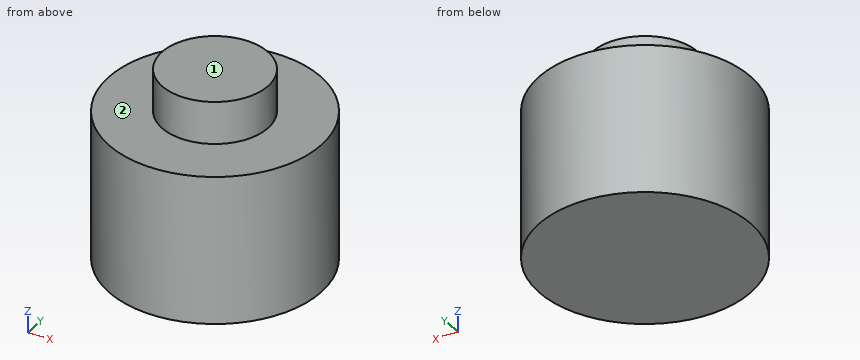
```python
from build123d import *

# Parameters (mm, degrees)
F1_R      = 25
F2_DEPTH  = 25
F2_FACE_R = 25
F3_DEPTH  = 10
F4_R      = 12.5
F5_DEPTH  = 10


with BuildPart() as f2:
    # F1 (on Top) → F2 (new body)
    with BuildSketch(Plane.XY):
        Circle(F1_R)
    extrude(amount=F2_DEPTH)

    # F2_face (on face) → F3 (join)
    with BuildSketch(Plane.XY.offset(25)):
        Circle(F2_FACE_R)
    extrude(amount=F3_DEPTH)

    # F4 (on offset) → F5 (join)
    with BuildSketch(Plane.XY.offset(35)):
        Circle(F4_R)
    extrude(amount=F5_DEPTH)


solid = f2.part
```
Geometry: final body of the model. Coordinates: model frame, mm. Face numbers are marked on the shaded views. A direction names the side the tool comes from. Coordinates: 2 decimals unless noted, no trailing zeros. Order: outer loops, then holes, each group sorted by start corner. A loop starts at its lowest first (then second) coordinate and runs counter-clockwise, first axis right, second up. Notation, with made-up numbers: M 0,82 L 30,82 A13 ccw 30,92 Z; hole C -0.5,70.25 d10. An arc over 180 degrees is marked long. Answer in a Markdown table with one row per item. Add a question column.
Q1. Section query D-D on y = 13.5. Return the cut outline in (x, z), and give its area (3 significant figures).
Q2. Contact query for flat-ended pins moving along their axis: P1, Ø4, axis at x = -4, z = 34, coming from the +Y side; P2, Ø10, axis at y = -19.5, z = 9.5, coming from the +X side; P3, Ø4, axis at x = 5, y = -15.5, coming from the -Z side; P4, Ø1.5, axis at y = -16, z = 6.5, coming from the -X side. Output: stop coordinate, or through.
Q3. Section query A-A on x = 0. Return the cut outline in (y, z).
Q4. Section query C-C on z = 6.5. Return the cut outline in (x, y), and give its area (3 significant figures).
Q5. Reachability of the marked faces 1 and 2 from +Z, -Z, +X, -X, +Y, -Y: full face, straight path, thin tool, end or side. Return the list, or none.
Q6. Line query: L1, parallel to Z at x = -12, y = -17; L2, parallel to X at y = -10.5, z = 4.5; L3, parallel to Y at x = -22, z = 33.5. Output: solid intervals per line, ascending.
Completed:
| question | item | result |
|---|---|---|
| 1 | outline | M -21.04,0 L 21.04,0 L 21.04,35 L -21.04,35 Z |
| 1 | area | 1,470 mm2 |
| 2 | P1 | stops at y = 24.92 |
| 2 | P2 | stops at x = 20.37 |
| 2 | P3 | stops at z = 0 |
| 2 | P4 | stops at x = -19.81 |
| 3 | outline | M -25,0 L 25,0 L 25,35 L 12.5,35 L 12.5,45 L -12.5,45 L -12.5,35 L -25,35 Z |
| 4 | outline | C 0,0 d50 |
| 4 | area | 1,960 mm2 |
| 5 | face 1 | +Z, +X, -X, +Y, -Y |
| 5 | face 2 | +Z |
| 6 | L1 | z = 0 to 35 |
| 6 | L2 | x = -22.69 to 22.69 |
| 6 | L3 | y = -11.87 to 11.87 |
